from build123d import *

# Parameters (mm, degrees)
BOSS_EXTRUDE1_DEPTH = 15
SKETCH2_R           = 4.5
CUT_EXTRUDE1_DEPTH  = 9
SKETCH3_R           = 2.75
CUT_EXTRUDE2_DEPTH  = 136.49768983
BOSS_EXTRUDE2_START = 65
BOSS_EXTRUDE2_DEPTH = 65
BOSS_EXTRUDE3_START = 22
BOSS_EXTRUDE3_DEPTH = 22
SKETCH6_R           = 2.5
CUT_EXTRUDE3_DEPTH  = 4


with BuildPart() as part:
    # Sketch1 → Boss-Extrude1 (new body)
    with BuildSketch(Plane(origin=(0, 0, 0), x_dir=(1, 0, 0), z_dir=(0, 1, 0))):
        with BuildLine():
            Line((-24.748737342, 24.748737342), (41.489469156, 90.986943839))
            ThreePointArc((41.489469156, 90.986943839), (92.387953251, 38.268343237), (93.674969976, -35))
            Line((93.674969976, -35), (0, -35))
            ThreePointArc((0, -35), (-32.335783638, -13.393920133), (-24.748737342, 24.748737342))
        make_face()
    extrude(amount=BOSS_EXTRUDE1_DEPTH)

    # Sketch2 → Cut-Extrude1 (cut)
    with BuildSketch(Plane(origin=(0, 15, 0), x_dir=(1, 0, 0), z_dir=(0, 1, 0))):
        with Locations(Location((0, 19, 0), (0, 0, 270))):
            Circle(SKETCH2_R)
        with Locations(Location((16.454482672, 9.5, 0), (0, 0, 270))):
            Circle(SKETCH2_R)
        with Locations(Location((16.454482672, -9.5, 0), (0, 0, 270))):
            Circle(SKETCH2_R)
        with Locations(Location((0, -19, 0), (0, 0, 270))):
            Circle(SKETCH2_R)
        with Locations(Location((-16.454482672, -9.5, 0), (0, 0, 270))):
            Circle(SKETCH2_R)
        with Locations(Location((-16.454482672, 9.5, 0), (0, 0, 270))):
            Circle(SKETCH2_R)
    extrude(amount=-CUT_EXTRUDE1_DEPTH, mode=Mode.SUBTRACT)

    # Sketch3 → Cut-Extrude2 (cut, through all)
    with BuildSketch(Plane(origin=(0, 6, 0), x_dir=(1, 0, 0), z_dir=(0, 1, 0))):
        with Locations(Location((0, 19, 0), (0, 0, 270))):
            Circle(SKETCH3_R)
        with Locations(Location((16.454482672, 9.5, 0), (0, 0, 270))):
            Circle(SKETCH3_R)
        with Locations(Location((16.454482672, -9.5, 0), (0, 0, 270))):
            Circle(SKETCH3_R)
        with Locations(Location((0, -19, 0), (0, 0, 270))):
            Circle(SKETCH3_R)
        with Locations(Location((-16.454482672, -9.5, 0), (0, 0, 270))):
            Circle(SKETCH3_R)
        with Locations(Location((-16.454482672, 9.5, 0), (0, 0, 270))):
            Circle(SKETCH3_R)
    extrude(amount=-CUT_EXTRUDE2_DEPTH, mode=Mode.SUBTRACT)

    # Sketch4 → Boss-Extrude2 (add)
    with BuildSketch(Plane.XZ.offset(BOSS_EXTRUDE2_START)):
        with BuildLine():
            Line((93.674969976, 35), (82.915619759, 35))
            ThreePointArc((82.915619759, 35), (83.149157926, -34.441508913), (33.881459656, -83.378934339))
            Line((33.881459656, -83.378934339), (41.489469156, -90.986943839))
            ThreePointArc((41.489469156, -90.986943839), (92.387953251, -38.268343237), (93.674969976, 35))
        make_face()
    extrude(amount=-BOSS_EXTRUDE2_DEPTH)

    # Sketch5 → Boss-Extrude3 (add)
    with BuildSketch(Plane.XZ.offset(BOSS_EXTRUDE3_START)):
        with BuildLine():
            Line((80.428539711, 23.5), (86.877787725, 23.5))
            ThreePointArc((86.877787725, 23.5), (85.091202872, 29.317012019), (82.915619759, 35))
            Line((82.915619759, 35), (76.428539711, 35))
            Line((76.428539711, 35), (76.428539711, 27.5))
            ThreePointArc((76.428539711, 27.5), (77.600112586, 24.671572875), (80.428539711, 23.5))
        make_face()
        with BuildLine():
            Line((34.597702223, -73.488575188), (29.294401364, -78.791876047))
            Line((29.294401364, -78.791876047), (33.881459656, -83.378934339))
            ThreePointArc((33.881459656, -83.378934339), (39.438308567, -80.898824573), (44.814863477, -78.048882193))
            Line((44.814863477, -78.048882193), (40.254556473, -73.488575188))
            ThreePointArc((40.254556473, -73.488575188), (37.426129348, -72.317002313), (34.597702223, -73.488575188))
        make_face()
    extrude(amount=-BOSS_EXTRUDE3_DEPTH)

    # Sketch6 → Cut-Extrude3 (cut)
    with BuildSketch(Plane.XZ.offset(22)):
        with Locations(Location((80.428539711, 27.5, 0), (0, 0, 270))):
            Circle(SKETCH6_R)
        with Locations(Location((37.426129348, -76.317002313, 0), (0, 0, 270))):
            Circle(SKETCH6_R)
    extrude(amount=-CUT_EXTRUDE3_DEPTH, mode=Mode.SUBTRACT)


solid = part.part
Work out the finished part from the listing and answer in its coordinate system (mm). A direction names the side the tool comes from. Give positions to 0.01 mm unless a question says otherwise; leave off trailing zeros. Loops run counter-clockwise (first coordinate to the right, second up) from the corner with the lowest first, then second, coordinate; pieces in that order, holes last. Notation, with made-up numbers: (58, -34.75) -> (106, -34.75) arc R8 cw to (106, -24.75) -> close; hole circle Ø1 at (64, 5.5). An arc over 180 degrees is marked (long way). Use a Markdown table: item, result. Add a question column.
1. Section C-C on x = 64 is taken. Determine the outline of the cut face in (y, z).
2. Section D-D on z = -62.5 is taken. Determine the outline of the cut face in (x, y), and give its area (3 significant figures).
3. Section B-B on y = -15 is taken. Determine the outline of the cut face in (x, z).
4. Flat-ended cylindrical pins translate along their axes: pin 1 Ø4 at (y, z) = (-14, -9) entering from +X; pin 2 Ø5 at (x, z) = (64, -13.5) entering from -Y; pin 3 Ø2 at (x, y) = (84.5, -12) entering from -Z (3 decimals). Find the tip coordinate at first contact, or state that the pin passes through.
5. For faces 1 (the flat face through (82, -22, 31)), 2 (the flat face through (61, 1, 35)), 3 (the flat face through (37, -18, -76)), 4 (the flat face through (19, 6, -8)), 5 (the flat face through (37, -22, -79)), determine the directions among +Z, -Z, +X, -X, +Y, -Y from which every point of the face is accessible in a straight line to the end or side of a thin tool.
6. Determine the mould class of faces 6 (the cylindrical face through (91.98, -25.56, -39.24)), 7 (the cylindrical face through (12.462, 10.563, 11.576)), 8 (the flat face through (42.567, -11.154, -75.801)) for opening direction Z: released by +Z, released by -Z, zero draft, split by the parting line, or undercut.
7. Section A-A on z = 19 is taken. Determine the outline of the cut face in (x, y).
8. Find the intervals of material crossed by probe 1 along X at (y, z) = (12.25, 9.5); probe 2 along Y at (x, z) = (-6, -12); probe 3 along X at (y, z) = (10, 9), in increasing order.
Results below:
| question | item | result |
|---|---|---|
| 1 | outline | (-65, -76.84) -> (15, -76.84) -> (15, 35) -> (0, 35) -> (0, -63.28) -> (-65, -63.28) -> close |
| 2 | outline | (13, 0) -> (64.76, 0) -> (64.76, -65) -> (78.06, -65) -> (78.06, 15) -> (13, 15) -> close |
| 2 | area | 1,840 mm^2 |
| 3 | outline | (29.29, -78.79) -> (41.49, -90.99) arc R100 ccw to (93.67, 35) -> (76.43, 35) -> (76.43, 27.5) arc R4 ccw to (80.43, 23.5) -> (86.88, 23.5) arc R90 cw to (44.81, -78.05) -> (40.25, -73.49) arc R4 ccw to (34.6, -73.49) -> close |
| 4 | pin 1 | stops at x = 99.75 |
| 4 | pin 2 | stops at y = 0 |
| 4 | pin 3 | stops at z = -55.025 |
| 5 | face 1 | -X, -Y |
| 5 | face 2 | +Z, +X, -X, +Y, -Y |
| 5 | face 3 | -Y |
| 5 | face 4 | +Y |
| 5 | face 5 | +Z, -X, -Y |
| 6 | face 6 | split by the parting line |
| 6 | face 7 | undercut |
| 6 | face 8 | released by +Z |
| 7 | outline | (-29.39, 0) -> (-2.75, 0) -> (-2.75, 6) -> (-4.5, 6) -> (-4.5, 15) -> (-29.39, 15) -> close; (2.75, 0) -> (87.97, 0) -> (87.97, -65) -> (98.18, -65) -> (98.18, 15) -> (4.5, 15) -> (4.5, 6) -> (2.75, 6) -> close |
| 8 | probe 1 | x = -33.69 to -20.95, -11.95 to 11.95, 20.95 to 99.55 |
| 8 | probe 2 | y = 0 to 15 |
| 8 | probe 3 | x = -33.82 to -20.93, -11.98 to 11.98, 20.93 to 99.59 |
